Could you check a few things on this model? Use its own coordinates, in mm. Face numbers are marked on the shaded views. Give positions to 0.01 mm unless a question says otherwise; leave off trailing zeros. Loops run counter-clockwise (first coordinate to the right, second up) from the corner with the lowest first, then second, coordinate; pieces in that order, holes last. Notation, with made-up numbers: (-33, 64) -> (-7, 64) arc R25 ccw to (-7, 93) -> close; hole circle Ø3 at (-39.75, -24). An arc over 180 degrees is marked (long way). Put each result on its own line as item: value.
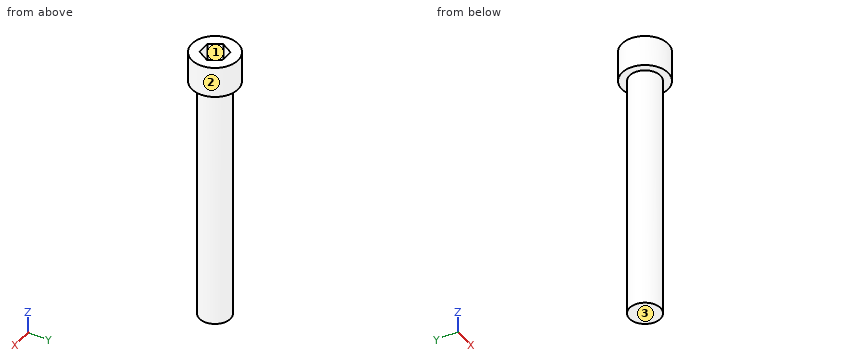
```python
from build123d import *

# Parameters (mm, degrees)
SKETCH1_R           = 3.175
BOSS_EXTRUDE1_DEPTH = 50.8
SKETCH2_R           = 4.7625
BOSS_EXTRUDE2_DEPTH = 6.35
CUT_EXTRUDE1_DEPTH  = 3.5814


with BuildPart() as part:
    # Sketch1 → Boss-Extrude1 (new body)
    with BuildSketch(Plane.XY):
        Circle(SKETCH1_R)
    extrude(amount=BOSS_EXTRUDE1_DEPTH)

    # Sketch2 → Boss-Extrude2 (add)
    with BuildSketch(Plane.XY.offset(50.8)):
        Circle(SKETCH2_R)
    extrude(amount=BOSS_EXTRUDE2_DEPTH)

    # Sketch3 → Cut-Extrude1 (cut)
    with BuildSketch(Plane.XY.offset(57.15)):
        Polygon((2.749630657, 0), (1.374815329, 2.38125), (-1.374815329, 2.38125), (-2.749630657, 0), (-1.374815329, -2.38125), (1.374815329, -2.38125), align=None)
    extrude(amount=-CUT_EXTRUDE1_DEPTH, mode=Mode.SUBTRACT)


solid = part.part
```
1. I need wall thicknesses on line 1 (Z direction, x = -3.5, y = -3); line 2 (Y direction, x = 0, z = 36) (3 decimals); line 3 (X direction, y = -0.25, z = 8). Which ranges of each line are inside material? Lowest first, please.
Recorded:
line 1: z = 50.8 to 57.15
line 2: y = -3.175 to 3.175
line 3: x = -3.17 to 3.17
2. Thinking about a two-plate mould opening in Y: for the marked faces 1, 2 and 3, which applies, pulls with the +Y half, pulls with the -Y half, needs draft (parallel to the pull), parting line crosses it, or undercut?
Recorded:
face 1: undercut
face 2: parting line crosses it
face 3: needs draft
3. I'm going to push flat-ended pins straight in: pin 1 (3 mm diameter, centred on x = 2, z = 10, fed in from +Y); pin 2 (5 mm diameter, centred on x = -2, y = -2, fed in from -Z); pin 3 (5 mm diameter, centred on y = -1, z = 12.5, fed in from +X) (3 decimals); pin 4 (5 mm diameter, centred on x = -3.5, z = 37, fed in from +Y). Where does each tip first touch, or does it pass through?
Recorded:
pin 1: stops at y = 3.14
pin 2: stops at z = 0
pin 3: stops at x = 3.175
pin 4: stops at y = 3.01
4. If we section it at B-B (y = 1.5): List the corners of the cut face in (x, z) for me.
Recorded:
outline: (-4.52, 50.8) -> (-2.8, 50.8) -> (-2.8, 0) -> (2.8, 0) -> (2.8, 50.8) -> (4.52, 50.8) -> (4.52, 57.15) -> (1.88, 57.15) -> (1.88, 53.57) -> (-1.88, 53.57) -> (-1.88, 57.15) -> (-4.52, 57.15) -> close
5. If we section it at C-C (z = 30): List the corners of the cut face in (x, y) for me (3 decimals), then the cut area to 3 significant figures.
Recorded:
outline: circle Ø6.35 at (0, 0)
area: 31.7 mm^2
